from build123d import *

# Parameters (mm, degrees)
SKETCH2_W                  = 254
SKETCH2_H                  = 101.6
RECTANGLE_EXTRUSION_DEPTH  = 12.7
SKETCH4_W                  = 12.7
SKETCH4_H                  = 12.7
FRONT_FACE_TABS_DEPTH      = 12.7
SKETCH6_R                  = 2.24536
TAB_CURVE_FRONT_BACK_DEPTH = 12.7
SKETCH7_W                  = 12.7
SKETCH7_H                  = 12.7
RIGHT_FACE_TABS_DEPTH      = 12.7
SKETCH8_R                  = 2.24536
TAB_CURVE_LEFT_RIGHT_DEPTH = 12.7


with BuildPart() as part:
    # Sketch2 → Rectangle Extrusion (new body)
    with BuildSketch(Plane(origin=(0, 0, 0), x_dir=(1, 0, 0), z_dir=(0, 1, 0))):
        Rectangle(SKETCH2_W, SKETCH2_H)
    extrude(amount=RECTANGLE_EXTRUSION_DEPTH)

    # Sketch4 → Front Face Tabs (add)
    with BuildSketch(Plane.XY.offset(50.8)):
        with Locations((-63.5, 6.35)):
            Rectangle(SKETCH4_W, SKETCH4_H)
        with Locations((63.5, 6.35)):
            Rectangle(SKETCH4_W, SKETCH4_H)
    front_face_tabs = extrude(amount=FRONT_FACE_TABS_DEPTH)

    # Mirror Rear Face Tabs: Front Face Tabs across plane
    add(front_face_tabs.mirror(Plane.XY))

    # Sketch6 → Tab Curve Front Back (cut)
    with BuildSketch(Plane(origin=(0, 12.7, 0), x_dir=(1, 0, 0), z_dir=(0, 1, 0))):
        with Locations((-71.4375, 52.3875)):
            Circle(SKETCH6_R)
        with Locations((-55.5625, 52.3875)):
            Circle(SKETCH6_R)
        with Locations((55.5625, 52.3875)):
            Circle(SKETCH6_R)
        with Locations((71.4375, 52.3875)):
            Circle(SKETCH6_R)
        with Locations((71.4375, -52.3875)):
            Circle(SKETCH6_R)
        with Locations((55.5625, -52.3875)):
            Circle(SKETCH6_R)
        with Locations((-55.5625, -52.3875)):
            Circle(SKETCH6_R)
        with Locations((-71.4375, -52.3875)):
            Circle(SKETCH6_R)
    extrude(amount=-TAB_CURVE_FRONT_BACK_DEPTH, mode=Mode.SUBTRACT)

    # Sketch7 → Right Face Tabs (add)
    with BuildSketch(Plane(origin=(127, 0, 0), x_dir=(0, 0, -1), z_dir=(1, 0, 0))):
        with Locations((-25.4, 6.35)):
            Rectangle(SKETCH7_W, SKETCH7_H)
        with Locations((25.4, 6.35)):
            Rectangle(SKETCH7_W, SKETCH7_H)
    right_face_tabs = extrude(amount=RIGHT_FACE_TABS_DEPTH)

    # Mirror Left Face Tabs: Right Face Tabs across plane
    add(right_face_tabs.mirror(Plane(origin=(0, 0, 0), x_dir=(0, 0, 1), z_dir=(1, 0, 0))))

    # Sketch8 → Tab Curve Left Right (cut)
    with BuildSketch(Plane(origin=(0, 12.7, 0), x_dir=(1, 0, 0), z_dir=(0, 1, 0))):
        with Locations((128.5875, 33.3375)):
            Circle(SKETCH8_R)
        with Locations((128.5875, 17.4625)):
            Circle(SKETCH8_R)
        with Locations((128.5875, -17.4625)):
            Circle(SKETCH8_R)
        with Locations((128.5875, -33.3375)):
            Circle(SKETCH8_R)
        with Locations((-128.5875, -33.3375)):
            Circle(SKETCH8_R)
        with Locations((-128.5875, -17.4625)):
            Circle(SKETCH8_R)
        with Locations((-128.5875, 17.4625)):
            Circle(SKETCH8_R)
        with Locations((-128.5875, 33.3375)):
            Circle(SKETCH8_R)
    extrude(amount=-TAB_CURVE_LEFT_RIGHT_DEPTH, mode=Mode.SUBTRACT)


solid = part.part
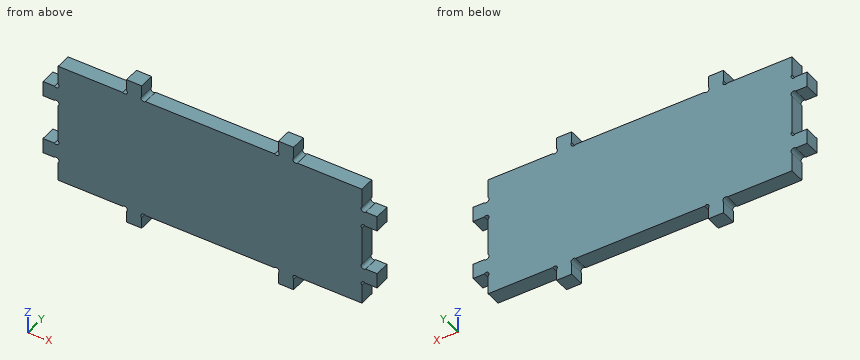
For this review, take the finished solid that the model builds, in its own axes (mm). Coordinates: 2 decimals unless noted, no trailing zeros. Loops run counter-clockwise (first coordinate to the right, second up) from the corner with the lowest first, then second, coordinate; pieces in that order, holes last. Notation, with made-up numbers: (20.5, 39) -> (74.5, 39) arc R24 cw to (74.5, 59) -> close; hole circle Ø11 at (21, 50.5). An arc over 180 degrees is marked (long way). Write each question's results on one line, items separated by ' | '.
Q1. For pin 1 Ø5 at (x, y) = (133, 7.5) entering from -Z; pin 2 Ø6.5 at (y, z) = (6, 39.5) entering from -X; pin 3 Ø7.5 at (x, y) = (134, 3.5) entering from +Z; pin 4 Ø6 at (x, z) = (43.5, -21.5) entering from -Y, all flat-tipped, find the tip position at first contact; note any pin that passes through.
Taken from the geometry:
pin 1: z = -31.75 | pin 2: x = -127 | pin 3: z = 31.75 | pin 4: y = 0
Q2. Add section A-A, the plane z = -1. State the section outline as (x, y) points.
Taken from the geometry:
outline: (-127, 0) -> (127, 0) -> (127, 12.7) -> (-127, 12.7) -> close
Q3. To check wall thickness, follow line 1 along X through (y, z) = (11.75, -54); line 2 along X through (y, z) = (4.5, -52.5); line 3 along X through (y, z) = (3.5, 48). State the ranges of each line that lie inside material, in increasing order. Write a range as [from, to].
Taken from the geometry:
line 1: [-69.85, -57.15], [57.15, 69.85] | line 2: [-69.19, -57.81], [57.81, 69.19] | line 3: [-127, 127]
Q4. Add section B-B, the plane x = -114. State the section outline as (y, z) points, then the cut area to 3 significant figures.
Taken from the geometry:
outline: (0, -50.8) -> (12.7, -50.8) -> (12.7, 50.8) -> (0, 50.8) -> close | area: 1,290 mm²
